Geometry check sheet. Reference: the model listing, model coordinates, mm. A direction names the side the tool comes from. Give positions to 0.01 mm unless a question says otherwise; leave off trailing zeros. Write each loop counter-clockwise with the first axis right and the second up, starting at its lowest first coordinate (ties: lowest second). Pieces come first, ordered by that corner, then holes.
(1) Cross-section at A-A (x = 6). Record the boundary of the cut face in (y, z), and give its area (3 significant figures).
(2) Thickness scan on line 1 along X through (y, z) = (8.25, 1.5); line 2 along X through (y, z) = (0.25, 1.3); line 3 along Y through (x, z) = (-6.75, 1.35). Record the ranges inside material, lowest first.
(3) Cross-section at B-B (x = -6.75). Record the boundary of the cut face in (y, z), and give its area (3 significant figures).
(4) Depth check by flat-ended pin: P1, Ø1, axis at x = -3.5, z = 1, coming from the -Y side; P2, Ø1.6, axis at x = 0, y = 0, coming from the +Z side. Enter the tip coordinate at first touch or a pass-through.
(5) Tool access check on faces 5 (the cylindrical face through (5.91, -8.11, 0.99)), 6 (the cylindrical face through (-9.575, -3.087, 0.986)), 7 (the cylindrical face through (-9.857, -1.894, 0.986)). Record the directions out of +Z, -Z, +X, -X, +Y, -Y that give a thin tool (end or side, any length) a straight path to the whole face; none if there is none.
(6) Mould release check, pull along Y, two halves, no side actions. Record for faces 1 (the cylindrical face through (0, -10, 1)), 2 (the cylindrical face through (-9.09, 4.3, 0.99)), 3 (the cylindrical face through (1.283, 9.978, 0.986)), 4 (the cylindrical face through (-8.482, 5.366, 0.986)): +Y half, -Y half, draft (parallel to the pull), parting line (faces both ways), or undercut.
```python
from build123d import *

# Parameters (mm, degrees)
F0_R     = 1
F1_DEPTH = 2


with BuildPart() as f1:
    # F0 (on Top) → F1 (new body)
    with BuildSketch(Plane.XY):
        with BuildLine():
            ThreePointArc((1.003907, 9.145063), (0.577673, 9.181846), (0.150189, 9.198774))
            ThreePointArc((0.150189, 9.198774), (-0.018265, 10.048606), (-0.466655, 10.789913))
            ThreePointArc((-0.466655, 10.789913), (-0.678138, 10.778689), (-0.889359, 10.763319))
            ThreePointArc((-0.889359, 10.763319), (-1.241303, 9.971659), (-1.301917, 9.107415))
            ThreePointArc((-1.301917, 9.107415), (-1.723908, 9.037043), (-2.142172, 8.947128))
            ThreePointArc((-2.142172, 8.947128), (-2.516678, 9.728368), (-3.135337, 10.334876))
            ThreePointArc((-3.135337, 10.334876), (-3.337384, 10.27141), (-3.538147, 10.203995))
            ThreePointArc((-3.538147, 10.203995), (-3.682156, 9.349681), (-3.525937, 8.497516))
            ThreePointArc((-3.525937, 8.497516), (-3.917169, 8.324409), (-4.299932, 8.133301))
            ThreePointArc((-4.299932, 8.133301), (-4.856958, 8.796861), (-5.607013, 9.23046))
            ThreePointArc((-5.607013, 9.23046), (-5.786929, 9.118742), (-5.96462, 9.003516))
            ThreePointArc((-5.96462, 9.003516), (-5.891646, 8.140229), (-5.528409, 7.353686))
            ThreePointArc((-5.528409, 7.353686), (-5.864301, 7.088722), (-6.187511, 6.808429))
            ThreePointArc((-6.187511, 6.808429), (-6.892059, 7.312615), (-7.726381, 7.546061))
            ThreePointArc((-7.726381, 7.546061), (-7.872861, 7.393109), (-8.016314, 7.237314))
            ThreePointArc((-8.016314, 7.237314), (-7.730941, 6.419296), (-7.183511, 5.747797))
            ThreePointArc((-7.183511, 5.747797), (-7.442956, 5.407624), (-7.686307, 5.055758))
            ThreePointArc((-7.686307, 5.055758), (-8.494105, 5.368891), (-9.360272, 5.387515))
            ThreePointArc((-9.360272, 5.387515), (-9.464112, 5.20294), (-9.564314, 5.016364))
            ThreePointArc((-9.564314, 5.016364), (-9.084474, 4.295015), (-8.387247, 3.780752))
            ThreePointArc((-8.387247, 3.780752), (-8.553944, 3.386746), (-8.702143, 2.985416))
            ThreePointArc((-8.702143, 2.985416), (-9.562436, 3.087819), (-10.406022, 2.890451))
            ThreePointArc((-10.406022, 2.890451), (-10.460698, 2.685851), (-10.511352, 2.480218))
            ThreePointArc((-10.511352, 2.480218), (-9.867195, 1.900862), (-9.063981, 1.57615))
            ThreePointArc((-9.063981, 1.57615), (-9.127455, 1.153066), (-9.171192, 0.727488))
            ThreePointArc((-9.171192, 0.727488), (-10.029924, 0.612728), (-10.797924, 0.21177))
            ThreePointArc((-10.797924, 0.21177), (-10.8, 0), (-10.797924, -0.21177))
            ThreePointArc((-10.797924, -0.21177), (-10.029924, -0.612728), (-9.171192, -0.727488))
            ThreePointArc((-9.171192, -0.727488), (-9.127455, -1.153066), (-9.063981, -1.57615))
            ThreePointArc((-9.063981, -1.57615), (-9.867195, -1.900862), (-10.511352, -2.480218))
            ThreePointArc((-10.511352, -2.480218), (-10.460698, -2.685851), (-10.406022, -2.890451))
            ThreePointArc((-10.406022, -2.890451), (-9.562436, -3.087819), (-8.702143, -2.985416))
            ThreePointArc((-8.702143, -2.985416), (-8.553944, -3.386746), (-8.387247, -3.780752))
            ThreePointArc((-8.387247, -3.780752), (-9.084474, -4.295015), (-9.564314, -5.016364))
            ThreePointArc((-9.564314, -5.016364), (-9.464112, -5.20294), (-9.360272, -5.387515))
            ThreePointArc((-9.360272, -5.387515), (-8.494105, -5.368891), (-7.686307, -5.055758))
            ThreePointArc((-7.686307, -5.055758), (-7.442956, -5.407624), (-7.183511, -5.747797))
            ThreePointArc((-7.183511, -5.747797), (-7.730941, -6.419296), (-8.016314, -7.237314))
            ThreePointArc((-8.016314, -7.237314), (-7.872861, -7.393109), (-7.726381, -7.546061))
            ThreePointArc((-7.726381, -7.546061), (-6.892059, -7.312615), (-6.187511, -6.808429))
            ThreePointArc((-6.187511, -6.808429), (-5.864301, -7.088722), (-5.528409, -7.353686))
            ThreePointArc((-5.528409, -7.353686), (-5.891646, -8.140229), (-5.96462, -9.003516))
            ThreePointArc((-5.96462, -9.003516), (-5.786929, -9.118742), (-5.607013, -9.23046))
            ThreePointArc((-5.607013, -9.23046), (-4.856958, -8.796861), (-4.299932, -8.133301))
            ThreePointArc((-4.299932, -8.133301), (-3.917169, -8.324409), (-3.525937, -8.497516))
            ThreePointArc((-3.525937, -8.497516), (-3.682156, -9.349681), (-3.538147, -10.203995))
            ThreePointArc((-3.538147, -10.203995), (-3.337384, -10.27141), (-3.135337, -10.334876))
            ThreePointArc((-3.135337, -10.334876), (-2.516678, -9.728368), (-2.142172, -8.947128))
            ThreePointArc((-2.142172, -8.947128), (-1.723908, -9.037043), (-1.301917, -9.107415))
            ThreePointArc((-1.301917, -9.107415), (-1.241303, -9.971659), (-0.889359, -10.763319))
            ThreePointArc((-0.889359, -10.763319), (-0.678138, -10.778689), (-0.466655, -10.789913))
            ThreePointArc((-0.466655, -10.789913), (-0.018265, -10.048606), (0.150189, -9.198774))
            ThreePointArc((0.150189, -9.198774), (0.577673, -9.181846), (1.003907, -9.145063))
            ThreePointArc((1.003907, -9.145063), (1.277545, -9.96708), (1.81531, -10.646344))
            ThreePointArc((1.81531, -10.646344), (2.023718, -10.608702), (2.231348, -10.566981))
            ThreePointArc((2.231348, -10.566981), (2.481296, -9.737453), (2.433113, -8.872427))
            ThreePointArc((2.433113, -8.872427), (2.842956, -8.74972), (3.246652, -8.608092))
            ThreePointArc((3.246652, -8.608092), (3.716121, -9.336234), (4.405917, -9.860421))
            ThreePointArc((4.405917, -9.860421), (4.598416, -9.772132), (4.789147, -9.680086))
            ThreePointArc((4.789147, -9.680086), (4.824947, -8.81446), (4.563155, -7.988593))
            ThreePointArc((4.563155, -7.988593), (4.929607, -7.767817), (5.285398, -7.530243))
            ThreePointArc((5.285398, -7.530243), (5.921199, -8.118757), (6.719684, -8.45493))
            ThreePointArc((6.719684, -8.45493), (6.884179, -8.321543), (7.046027, -8.184956))
            ThreePointArc((7.046027, -8.184956), (6.865429, -7.337622), (6.406477, -6.602806))
            ThreePointArc((6.406477, -6.602806), (6.706511, -6.297833), (6.992043, -5.979242))
            ThreePointArc((6.992043, -5.979242), (7.754226, -6.391149), (8.611228, -6.518186))
            ThreePointArc((8.611228, -6.518186), (8.737384, -6.348081), (8.860179, -6.175535))
            ThreePointArc((8.860179, -6.175535), (8.474532, -5.399734), (7.847257, -4.802141))
            ThreePointArc((7.847257, -4.802141), (8.062021, -4.432134), (8.259352, -4.052543))
            ThreePointArc((8.259352, -4.052543), (9.100027, -4.261962), (9.961698, -4.17188))
            ThreePointArc((9.961698, -4.17188), (10.041586, -3.975745), (10.117613, -3.778082))
            ThreePointArc((10.117613, -3.778082), (9.551148, -3.122561), (8.794965, -2.699739))
            ThreePointArc((8.794965, -2.699739), (8.910965, -2.287947), (9.007696, -1.871207))
            ThreePointArc((9.007696, -1.871207), (9.87404, -1.86498), (10.686237, -1.563439))
            ThreePointArc((10.686237, -1.563439), (10.714839, -1.353599), (10.739321, -1.143239))
            ThreePointArc((10.739321, -1.143239), (10.02763, -0.649186), (9.190053, -0.427703))
            ThreePointArc((9.190053, -0.427703), (9.2, 0), (9.190053, 0.427703))
            ThreePointArc((9.190053, 0.427703), (10.02763, 0.649186), (10.739321, 1.143239))
            ThreePointArc((10.739321, 1.143239), (10.714839, 1.353599), (10.686237, 1.563439))
            ThreePointArc((10.686237, 1.563439), (9.87404, 1.86498), (9.007696, 1.871207))
            ThreePointArc((9.007696, 1.871207), (8.910965, 2.287947), (8.794965, 2.699739))
            ThreePointArc((8.794965, 2.699739), (9.551148, 3.122561), (10.117613, 3.778082))
            ThreePointArc((10.117613, 3.778082), (10.041586, 3.975745), (9.961698, 4.17188))
            ThreePointArc((9.961698, 4.17188), (9.100027, 4.261962), (8.259352, 4.052543))
            ThreePointArc((8.259352, 4.052543), (8.062021, 4.432134), (7.847257, 4.802141))
            ThreePointArc((7.847257, 4.802141), (8.474532, 5.399734), (8.860179, 6.175535))
            ThreePointArc((8.860179, 6.175535), (8.737384, 6.348081), (8.611228, 6.518186))
            ThreePointArc((8.611228, 6.518186), (7.754226, 6.391149), (6.992043, 5.979242))
            ThreePointArc((6.992043, 5.979242), (6.706511, 6.297833), (6.406477, 6.602806))
            ThreePointArc((6.406477, 6.602806), (6.865429, 7.337622), (7.046027, 8.184956))
            ThreePointArc((7.046027, 8.184956), (6.884179, 8.321543), (6.719684, 8.45493))
            ThreePointArc((6.719684, 8.45493), (5.921199, 8.118757), (5.285398, 7.530243))
            ThreePointArc((5.285398, 7.530243), (4.929607, 7.767817), (4.563155, 7.988593))
            ThreePointArc((4.563155, 7.988593), (4.824947, 8.81446), (4.789147, 9.680086))
            ThreePointArc((4.789147, 9.680086), (4.598416, 9.772132), (4.405917, 9.860421))
            ThreePointArc((4.405917, 9.860421), (3.716121, 9.336234), (3.246652, 8.608092))
            ThreePointArc((3.246652, 8.608092), (2.842956, 8.74972), (2.433113, 8.872427))
            ThreePointArc((2.433113, 8.872427), (2.481296, 9.737453), (2.231348, 10.566981))
            ThreePointArc((2.231348, 10.566981), (2.023718, 10.608702), (1.81531, 10.646344))
            ThreePointArc((1.81531, 10.646344), (1.277545, 9.96708), (1.003907, 9.145063))
        make_face()
        Circle(F0_R, mode=Mode.SUBTRACT)
    extrude(amount=F1_DEPTH)


solid = f1.part
```
Reply:
1. outline: (-8.17, 0) - (8.17, 0) - (8.17, 2) - (-8.17, 2) - close
1. area: 32.7 mm2
2. line 1: x = -5.92 to -4.37, -4.07 to 4.68, 6.15 to 6.97
2. line 2: x = -10.75 to -0.97, 0.97 to 9.2
2. line 3: y = -7.24 to 7.24
3. outline: (-7.24, 0) - (7.24, 0) - (7.24, 2) - (-7.24, 2) - close
3. area: 29.0 mm2
4. P1: stops at y = -10.33
4. P2: passes through
5. face 5: +Z, -Z, -Y
5. face 6: +Z, -Z
5. face 7: +Z, -Z, -X
6. face 1: -Y half
6. face 2: undercut
6. face 3: +Y half
6. face 4: undercut
